For this review, take the finished solid that the model builds, in its own axes (mm). Face numbers are marked on the shaded views. A direction names the side the tool comes from. Coordinates: 2 decimals unless noted, no trailing zeros. Loops run counter-clockwise (first coordinate to the right, second up) from the corner with the lowest first, then second, coordinate; pieces in that order, holes last. Notation, with made-up numbers: (4, -15.75) - (25, -15.75) arc R6 cw to (25, -7.75) - close; hole circle Ø6 at (33, 85.25). An arc over 180 degrees is marked (long way). Answer as a JSON object with one key per item and string values. Group by question number.
Item 1: We need section A-A (z = 44.5). Give the boundary of the cut face in (x, y), then the cut area to 3 significant figures.
Item 2: Clearance check with flat-ended pins moving along their axes: pin 1 (8 mm diameter, centred on x = -83.5, y = 7, fed in from +Z); pin 2 (6 mm diameter, centred on x = -96.5, y = 4.5, fed in from +Z); pin 3 (1 mm diameter, centred on x = -78, y = 10.5, fed in from -Z). State where each tip first meets the part, or that it passes through.
Item 3: We need section D-D (y = 10). Give the boundary of the cut face in (x, z).
Item 4: Tool access review of the marked faces 1, 2 and 3: name each direction out of +Z, -Z, +X, -X, +Y, -Y from which nothing blocks a thin tool from reaching the whole face with its end or side.
Item 5: We need section B-B (y = 7.5). Give the boundary of the cut face in (x, z), then the cut area to 3 significant figures.
Item 6: We need section C-C (x = -71). Give the boundary of the cut face in (y, z), then the cut area to 3 significant figures.
Item 7: To check wall thickness, follow line 1 (Y direction, x = -97, z = 39); line 2 (Z direction, x = -84, y = 13.5); line 3 (Z direction, x = -73.5, y = 2) (3 decimals). State the ranges of each line that lie inside material, in increasing order.
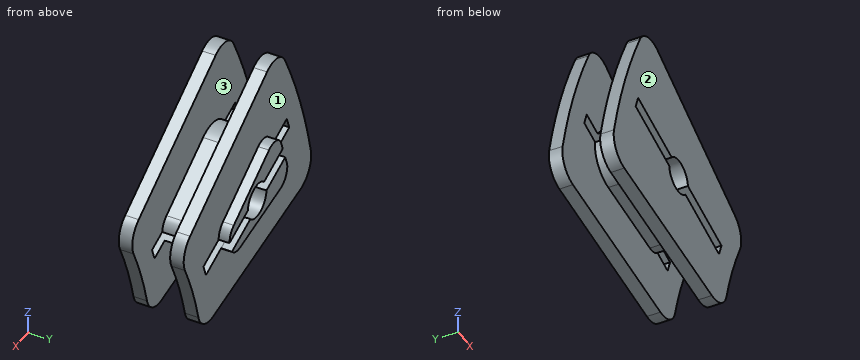
from build123d import *

# Parameters (mm, degrees)
BOSS_EXTRUDE1_DEPTH = 2.5
BOSS_EXTRUDE2_DEPTH = 7
CUT_EXTRUDE1_DEPTH  = 120.106847206
BOSS_EXTRUDE3_START = 2
BOSS_EXTRUDE3_DEPTH = 2


with BuildPart() as part:
    # Sketch1 → Boss-Extrude1 (new body)
    with BuildSketch(Plane(origin=(0, 0, 0), x_dir=(1, 0, 0), z_dir=(0, 1, 0))):
        with BuildLine():
            Line((-72.307015928, -13.524843261), (-102.896359968, -18.918569937))
            ThreePointArc((-102.896359968, -18.918569937), (-105.867796955, -20.867043845), (-106.499308602, -24.363782522))
            ThreePointArc((-106.499308602, -24.363782522), (-102.726730434, -37.092873959), (-97.434590717, -49.268890224))
            ThreePointArc((-97.434590717, -49.268890224), (-94.703164434, -51.541619594), (-91.174456756, -51.124234325))
            Line((-91.174456756, -51.124234325), (-64.274639058, -35.593617336))
            ThreePointArc((-64.274639058, -35.593617336), (-62.224627836, -33.023116562), (-62.470083693, -29.74443212))
            ThreePointArc((-62.470083693, -29.74443212), (-65.139025602, -23.412068226), (-67.164862535, -16.845633263))
            ThreePointArc((-67.164862535, -16.845633263), (-69.084330175, -14.176239282), (-72.307015928, -13.524843261))
        make_face()
    boss_extrude1 = extrude(amount=BOSS_EXTRUDE1_DEPTH)

    # Sketch2 → Boss-Extrude2 (add)
    with BuildSketch(Plane(origin=(0, 2.5, 0), x_dir=(1, 0, 0), z_dir=(0, 1, 0))):
        with BuildLine():
            Line((-75.996588964, -24.219866543), (-90.54428362, -26.785017618))
            ThreePointArc((-90.54428362, -26.785017618), (-94.837750272, -34.221520002), (-86.76867241, -37.158424161))
            Line((-86.76867241, -37.158424161), (-73.975644431, -29.772366014))
            ThreePointArc((-73.975644431, -29.772366014), (-72.656566568, -26.148229372), (-75.996588964, -24.219866543))
        make_face()
    extrude(amount=BOSS_EXTRUDE2_DEPTH)

    # Mirror1: Boss-Extrude1 across plane
    add(boss_extrude1.mirror(Plane.ZX.offset(6)))

    # Sketch4 → Cut-Extrude1 (cut, through all)
    with BuildSketch(Plane(origin=(0, 12, 0), x_dir=(1, 0, 0), z_dir=(0, 1, 0))):
        with BuildLine():
            Line((-98.925638819, -34.379167538), (-87.179481059, -30.103915746))
            ThreePointArc((-87.179481059, -30.103915746), (-85.044443484, -27.198470075), (-81.541325335, -28.051794886))
            Line((-81.541325335, -28.051794886), (-69.795167575, -23.776543095))
            Line((-69.795167575, -23.776543095), (-68.940117216, -26.125774647))
            Line((-68.940117216, -26.125774647), (-80.686274976, -30.401026438))
            ThreePointArc((-80.686274976, -30.401026438), (-82.821312552, -33.30647211), (-86.324430701, -32.453147298))
            Line((-86.324430701, -32.453147298), (-98.070588461, -36.72839909))
            Line((-98.070588461, -36.72839909), (-98.925638819, -34.379167538))
        make_face()
    extrude(amount=-CUT_EXTRUDE1_DEPTH, mode=Mode.SUBTRACT)

    # Sketch5 → Boss-Extrude3 (add)
    with BuildSketch(Plane(origin=(0, 12, 0), x_dir=(1, 0, 0), z_dir=(0, 1, 0)).offset(BOSS_EXTRUDE3_START)):
        with BuildLine():
            Line((-88.070170969, -37.828843014), (-75.758777587, -30.720856731))
            ThreePointArc((-75.758777587, -30.720856731), (-74.645598026, -29.596311171), (-74.25939673, -28.061834057))
            Line((-74.25939673, -28.061834057), (-80.686274976, -30.401026438))
            ThreePointArc((-80.686274976, -30.401026438), (-82.821312552, -33.30647211), (-86.324430701, -32.453147298))
            Line((-86.324430701, -32.453147298), (-92.880168291, -34.839240645))
            Line((-92.880168291, -34.839240645), (-92.238880522, -36.601164309))
            ThreePointArc((-92.238880522, -36.601164309), (-90.417678642, -38.108566439), (-88.070170969, -37.828843014))
        make_face()
        with BuildLine():
            Line((-77.97222629, -24.6394564), (-91.97222629, -27.108034129))
            ThreePointArc((-91.97222629, -27.108034129), (-93.95032425, -28.4027024), (-94.376506418, -30.728085429))
            Line((-94.376506418, -30.728085429), (-93.735218649, -32.490009093))
            Line((-93.735218649, -32.490009093), (-87.179481059, -30.103915746))
            ThreePointArc((-87.179481059, -30.103915746), (-85.044443484, -27.198470075), (-81.541325335, -28.051794886))
            Line((-81.541325335, -28.051794886), (-75.114447088, -25.712602505))
            ThreePointArc((-75.114447088, -25.712602505), (-76.396637321, -24.785370248), (-77.97222629, -24.6394564))
        make_face()
    extrude(amount=-BOSS_EXTRUDE3_DEPTH)


solid = part.part
Check sheet entries:
{
 "1": {"outline": "(-99.72, 0) - (-79.7, 0) - (-79.7, 2.5) - (-99.72, 2.5) - close; (-99.72, 9.5) - (-79.7, 9.5) - (-79.7, 12) - (-99.72, 12) - close", "area": "100 mm2"},
 "2": {"pin 1": "stops at z = 48.5", "pin 2": "stops at z = 51.65", "pin 3": "stops at z = 14.44"},
 "3": {"outline": "(-106.5, 24.36) arc R4.5 ccw to (-102.9, 18.92) - (-72.31, 13.52) arc R4.5 ccw to (-67.16, 16.85) arc R69 cw to (-62.47, 29.74) arc R4.5 ccw to (-64.27, 35.59) - (-91.17, 51.12) arc R4.5 ccw to (-97.43, 49.27) arc R109 ccw to start; hole (-98.93, 34.38) - (-87.18, 30.1) arc R3.25 ccw to (-81.54, 28.05) - (-69.8, 23.78) - (-68.94, 26.13) - (-80.69, 30.4) arc R3.25 ccw to (-86.32, 32.45) - (-98.07, 36.73) - close"},
 "4": {"face 1": "+Y", "face 2": "+Z, -Z, +X, -X, -Y", "face 3": "none"},
 "5": {"outline": "(-95.13, 33) arc R5.6 ccw to (-90.54, 26.79) - (-76, 24.22) arc R3 ccw to (-73.34, 25.07) - (-81.54, 28.05) arc R3.25 cw to (-87.18, 30.1) - close; (-94.28, 35.35) - (-86.32, 32.45) arc R3.25 cw to (-80.69, 30.4) - (-72.49, 27.42) arc R3 ccw to (-73.98, 29.77) - (-86.77, 37.16) arc R5.6 ccw to start", "area": "118 mm2"},
 "6": {"outline": "(0, 13.49) - (2.5, 13.49) - (2.5, 24.22) - (0, 24.22) - close; (0, 26.88) - (2.5, 26.88) - (2.5, 39.48) - (0, 39.48) - close; (9.5, 13.49) - (12, 13.49) - (12, 24.22) - (9.5, 24.22) - close; (9.5, 26.88) - (12, 26.88) - (12, 39.48) - (9.5, 39.48) - close", "area": "117 mm2"},
 "7": {"line 1": "y = 0 to 2.5, 9.5 to 12", "line 2": "z = 25.7 to 27, 33.5 to 35.48", "line 3": "z = 13.735 to 25.125, 27.785 to 40.92"}
}
